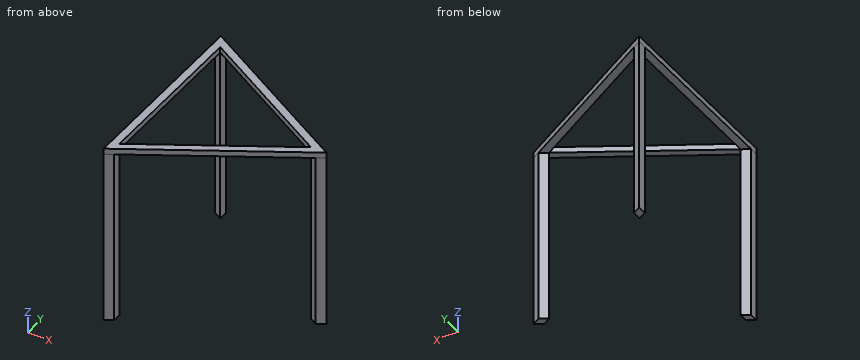
from build123d import *

# Parameters (mm, degrees)
F1_DEPTH = 5.08
F3_DEPTH = 152.4


with BuildPart() as f1:
    # F0 (on Top) → F1 (new body)
    with BuildSketch(Plane.XY):
        Polygon((95.243512, 1.311164), (-48.757257, 81.827719), (-46.486255, -83.138883), align=None)
        Polygon((-41.782549, 70.00239), (81.887859, 0.853349), (-39.832171, -71.673846), align=None, mode=Mode.SUBTRACT)
    extrude(amount=F1_DEPTH)

    # F2 (on face) → F3 (join)
    with BuildSketch(Plane(origin=(0, 0, 0), x_dir=(1, 0, 0), z_dir=(0, 0, -1))):
        Polygon((-41.782549, -77.927882), (-41.782549, -70.00239), (-48.647305, -73.840749), (-48.757257, -81.827719), align=None)
        Polygon((88.245812, 2.858434), (81.887859, -0.853349), (88.749803, -4.942055), (95.243512, -1.311164), align=None)
        Polygon((-46.588666, 75.69972), (-39.832171, 71.673846), (-39.832171, 79.17403), (-46.486255, 83.138883), align=None)
    extrude(amount=F3_DEPTH)


solid = f1.part
Design review of the part built by this model. Coordinates are the model's own, in mm. Give positions to 0.01 mm unless a question says otherwise; leave off trailing zeros. Order: outer loops, then holes, each group sorted by start corner. A loop starts at its lowest first (then second) coordinate and runs counter-clockwise, first axis right, second up. Notation, with made-up numbers: (51.5, 47) - (70.5, 47) arc R6 ccw to (70.5, 53) - close; hole circle Ø9 at (-23.5, 40). An arc over 180 degrees is marked (long way). Write item = value, one per line. Start each with the question number.
Q1. To check wall thickness, follow L1, parallel to Z at x = 55.5, y = 23; L2, parallel to X at y = 71, z = -48.5. State the ranges of each line that lie inside material, in increasing order. Write a range as from..to.
Q2. We need section C-C on x = 72. State the section outline as (y, z) points.
Q3. We need section B-B on z = -140. State the section outline as (x, y) points, plus the area to 3 significant figures.
Q4. We need section A-A on y = 67. State the section outline as (x, z) points, plus the area to 3 significant figures.
Q5. Clearance check with flat-ended pins moving along their axes: pin 1 Ø8 at (y, z) = (-4.5, -48.5) entering from +X; pin 2 Ø4 at (y, z) = (74.5, -49) entering from +X; pin 3 Ø24.5 at (x, y) = (-1, 47) entering from -Z. State where each tip first meets the part, or that it passes through.
Working result:
q1.L1 = 0..5.08
q1.L2 = -43.57..-41.78
q2.outline = (-12.54, 0) - (-5.04, 0) - (-5.04, 5.08) - (-12.54, 5.08) - close; (6.38, 0) - (14.31, 0) - (14.31, 5.08) - (6.38, 5.08) - close
q3.outline = (-48.76, 81.83) - (-48.65, 73.84) - (-41.78, 70) - (-41.78, 77.93) - close; (-46.59, -75.7) - (-46.49, -83.14) - (-39.83, -79.17) - (-39.83, -71.67) - close; (81.89, 0.85) - (88.25, -2.86) - (95.24, 1.31) - (88.75, 4.94) - close
q3.area = 157 mm²
q4.outline = (-48.55, 0) - (-41.74, 0) - (-41.74, 5.08) - (-48.55, 5.08) - close; (-36.41, 0) - (-22.24, 0) - (-22.24, 5.08) - (-36.41, 5.08) - close
q4.area = 107 mm²
q5.pin_1 = 92.2
q5.pin_2 = -41.78
q5.pin_3 = 0
